```python
from build123d import *

# Parameters (mm, degrees)
SKETCH1_R          = 73.3072
SKETCH1_R_2        = 71.3072
EXTRUDE1_DEPTH     = 66.04
EXTRUDE2_START     = 24.511
SKETCH2_R          = 127
SKETCH2_R_2        = 71.3072
EXTRUDE2_DEPTH     = 24.511
CUT_EXTRUDE1_REACH = 203.14
SKETCH3_R          = 4.2
CIRPATTERN1_COUNT  = 24
EXTRUDE3_START     = -2
SKETCH4_R          = 73.3072
SKETCH4_R_2        = 25.4
EXTRUDE3_DEPTH     = 2
EXTRUDE5_START     = -5
SKETCH8_R          = 29.21
SKETCH8_R_2        = 25.4
EXTRUDE5_DEPTH     = 5


with BuildPart() as part:
    # Sketch1 → Extrude1 (new body)
    with BuildSketch(Plane.XY):
        Circle(SKETCH1_R)
        Circle(SKETCH1_R_2, mode=Mode.SUBTRACT)
    extrude(amount=-EXTRUDE1_DEPTH)

    # Sketch2 → Extrude2 (add)
    with BuildSketch(Plane.XY.offset(EXTRUDE2_START)):
        Circle(SKETCH2_R)
        Circle(SKETCH2_R_2, mode=Mode.SUBTRACT)
    extrude(amount=-EXTRUDE2_DEPTH)

    # Sketch3 → Cut-Extrude1 (cut, up to next)
    with BuildSketch(Plane.XY.offset(24.511), mode=Mode.PRIVATE) as cut_extrude1_sk1:
        with Locations((15.131327149, -114.933840422)):
            Circle(SKETCH3_R)
    cut_extrude1_tool1 = extrude(cut_extrude1_sk1.sketch, amount=-CUT_EXTRUDE1_REACH, mode=Mode.PRIVATE) & part.part
    cut_extrude1 = cut_extrude1_tool1.solids().sort_by_distance((15.131327, -114.93384, 24.511))[0]
    add(cut_extrude1, mode=Mode.SUBTRACT)

    # CirPattern1: Cut-Extrude1 ×24 about axis
    cirpattern1_axis = Axis((0, 0, 0), (0, 0, 1))
    for i in range(1, CIRPATTERN1_COUNT):
        add(cut_extrude1.rotate(cirpattern1_axis, i * 360 / CIRPATTERN1_COUNT), mode=Mode.SUBTRACT)

    # Sketch4 → Extrude3 (add)
    with BuildSketch(Plane(origin=(0, 0, -66.04), x_dir=(-1, 0, 0), z_dir=(0, 0, -1)).offset(EXTRUDE3_START)):
        with Locations(Location((0, 0, 0), (0, 0, 180))):
            Circle(SKETCH4_R)
        Circle(SKETCH4_R_2, mode=Mode.SUBTRACT)
    extrude(amount=EXTRUDE3_DEPTH)

    # Sketch8 → Extrude5 (add)
    with BuildSketch(Plane(origin=(0, 0, -66.04), x_dir=(-1, 0, 0), z_dir=(0, 0, -1)).offset(EXTRUDE5_START)):
        Circle(SKETCH8_R)
        Circle(SKETCH8_R_2, mode=Mode.SUBTRACT)
    extrude(amount=EXTRUDE5_DEPTH)

    # Sketch9 → Cut-Revolve1 (revolve, cut)
    with BuildSketch(Plane(origin=(0, 0, 0), x_dir=(1, 0, 0), z_dir=(0, 1, 0)), mode=Mode.PRIVATE) as cut_revolve1_sk:
        Polygon((-29.145718757, 61.04), (-25.4, 66.04), (-25.4, 61.04), align=None)
    revolve(cut_revolve1_sk.sketch.rotate(Axis((0, 0, 0), (0, 0, -1)), 180), axis=Axis((0, 0, 0), (0, 0, -1)), mode=Mode.SUBTRACT)


solid = part.part
```
Here's how the part is built. I have some questions about the finished solid (model axes, mm). A direction names the side the tool comes from. Give positions to 0.01 mm unless a question says otherwise; leave off trailing zeros. Loops run counter-clockwise (first coordinate to the right, second up) from the corner with the lowest first, then second, coordinate; pieces in that order, holes last. Notation, with made-up numbers: (82, 73.25) -> (88, 73.25) arc R7 ccw to (88, 85.25) -> close; hole circle Ø5 at (-26, -18.5). An arc over 180 degrees is marked (long way). Use one line per item in the form item = value. Start each with the question number.
1) For P1, Ø10, axis at x = 28, y = -76.5, coming from the -Z side; P2, Ø6.5, axis at x = -114.93, y = -15.13, coming from the -Z side; P3, Ø1.5, axis at x = 2, z = 10, coming from the +Y side; P4, Ø6, axis at y = 45.5, z = -41.5, coming from the -X side, each with a flat end and sliding along its axis, tell me the tip position at first contact or that it passes through.
2) Which directions (+Z, -Z, +X, -X, +Y, -Y) give clear straight access to the entire face, cutting with the end or side of a thin tool? Please do faces 4 (the face through (-88.64, 68.01, 12.43)), 5 (the face through (31, -1, -64.04)).
3) Please list where these lines run through material, in increasing order: line 1 along Y through (x, z) = (-3, -46.5); line 2 along X through (y, z) = (-44.5, 10); line 3 along Z through (x, y) = (7.5, 106.5).
4) Imagine slicing it at D-D (y = 35). Please give me the cut outline in (x, z).
5) Imagine slicing it at A-A (x = 0). Please give me the cut outline in (y, z).
6) Thinking about a two-plate mould opening in Y: for faces 1 (the face through (-27.53, -123.98, 12.43)), 2 (the face through (55, -55, 0)), 3 (the face through (-48, 105, 12)), which applies, +Y half, -Y half, draft (parallel to the pull), parting line (faces both ways), or undercut?
7) Imagine slicing it at C-C (z = -34). Please give me the cut outline in (x, y).
Check values:
q1.P1 = 0
q1.P2 = through
q1.P3 = 126.99
q1.P4 = -59.73
q2.face_4 = +Z, -Z
q2.face_5 = +Z
q3.line_1 = -73.25 to -71.24, 71.24 to 73.25
q3.line_2 = -118.95 to -111.3, -102.9 to -55.72, 55.72 to 102.9, 111.3 to 118.95
q3.line_3 = 0 to 24.51
q4.outline = (-122.08, 0) -> (-64.41, 0) -> (-64.41, -66.04) -> (64.41, -66.04) -> (64.41, 0) -> (122.08, 0) -> (122.08, 24.51) -> (62.13, 24.51) -> (62.13, -64.04) -> (-62.13, -64.04) -> (-62.13, 24.51) -> (-122.08, 24.51) -> close
q5.outline = (-127, 0) -> (-73.31, 0) -> (-73.31, -66.04) -> (-25.4, -66.04) -> (-29.15, -61.04) -> (-29.21, -61.04) -> (-29.21, -64.04) -> (-71.31, -64.04) -> (-71.31, 24.51) -> (-127, 24.51) -> close; (25.4, -66.04) -> (73.31, -66.04) -> (73.31, 0) -> (127, 0) -> (127, 24.51) -> (71.31, 24.51) -> (71.31, -64.04) -> (29.21, -64.04) -> (29.21, -61.04) -> (29.15, -61.04) -> close
q6.face_1 = parting line
q6.face_2 = draft
q6.face_3 = undercut
q7.outline = circle Ø146.61 at (0, 0); hole circle Ø142.61 at (0, 0)
